Read the model definition and answer for the solid it produces. Units are mm, in the model's axes. Face numbers are marked on the shaded views. A direction names the side the tool comes from. Coordinates: 2 decimals unless noted, no trailing zeros. Loops run counter-clockwise (first coordinate to the right, second up) from the corner with the lowest first, then second, coordinate; pieces in that order, holes last. Notation, with made-up numbers: (80.25, 26) -> (109.25, 26) arc R22 cw to (109.25, 53) -> close; hole circle Ø3 at (85.5, -27). An arc over 180 degrees is marked (long way). Answer as CSV lines item,"result".
Autodesk Inventor part; units mm, degrees
ref_plane "YZ Plane" through (0, 0, 0) normal (1, 0, 0) x (0, 1, 0)
ref_plane "XZ Plane" through (0, 0, 0) normal (0, 1, 0) x (-1, 0, 0)
ref_plane "XY Plane" through (0, 0, 0) normal (0, 0, 1) x (1, 0, 0)
sketch "Sketch1" plane through (0, 0, 0) normal (0, 0, 1) x (1, 0, 0)
  circle A0 centre (0, 0) radius 19
  dimension "d0" = 38
extrude "Base_Shell" add sketch "Sketch1" along normal mid plane 132
sketch "Sketch2" plane through (0, 0, 66) normal (0, 0, 1) x (1, 0, 0)
  circle A0 centre (0, 0) radius 8.75
  dimension "d3" = 17.5
extrude "Terminal_Shell" add sketch "Sketch2" along normal blind 3.8
sketch "Sketch3" plane through (0, 0, 69.8) normal (0, 0, 1) x (1, 0, 0)
  circle A0 centre (0, 0) radius 7.75
  dimension "d6" = 15.5
extrude "Terminal" add sketch "Sketch3" along normal blind 3
sketch "Sketch4" plane through (0, 0, 72.8) normal (0, 0, 1) x (1, 0, 0)
  circle A0 centre (0, 0) radius 2.5
  dimension "d9" = 5
extrude "M5_Terminal_Screw_hole" cut sketch "Sketch4" against normal blind 5
mirror "Mirror1" about plane through (0, 0, 0) normal (0, 0, 1) of "Terminal_Shell", "Terminal", "M5_Terminal_Screw_hole"
equation "\"d1\" = 3.47368 * d0"
equation "\"d3\" = 0.460526 * d0"
equation "\"d4\" = 0.1 * d0"
equation "\"d6\" = 0.407895 * d0"
equation "\"d7\" = 0.0789474 * d0"
equation "\"d9\" = 0.131579 * d0"
equation "\"d10\" = d9"
properties part number "38120s-10Ah" material "Nickel-Copper Alloy 400"
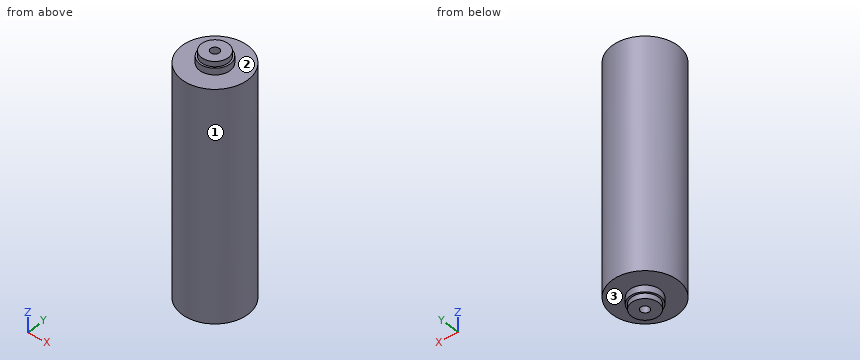
Q1. A cutting plane is placed at C-C, the plane z = -44. Write down the section's boundary in (x, y).
Results:
outline,"circle Ø38 at (0, 0)"
Q2. A cutting plane is placed at D-D, the plane y = -12. Write down the section's boundary in (x, z).
Results:
outline,"(-14.73, -66) -> (14.73, -66) -> (14.73, 66) -> (-14.73, 66) -> close"
Q3. A cutting plane is placed at A-A, the plane x = 0. Write down the section's boundary in (y, z), and give its area (3 significant figures).
Results:
outline,"(-19, -66) -> (-8.75, -66) -> (-8.75, -69.8) -> (-7.75, -69.8) -> (-7.75, -72.8) -> (-2.5, -72.8) -> (-2.5, -67.8) -> (2.5, -67.8) -> (2.5, -72.8) -> (7.75, -72.8) -> (7.75, -69.8) -> (8.75, -69.8) -> (8.75, -66) -> (19, -66) -> (19, 66) -> (8.75, 66) -> (8.75, 69.8) -> (7.75, 69.8) -> (7.75, 72.8) -> (2.5, 72.8) -> (2.5, 67.8) -> (-2.5, 67.8) -> (-2.5, 72.8) -> (-7.75, 72.8) -> (-7.75, 69.8) -> (-8.75, 69.8) -> (-8.75, 66) -> (-19, 66) -> close"
area,"5,190 mm²"
Q4. Given pin 1 Ø4 at (x, y) = (0, 0) entering from -Z; pin 2 Ø6 at (x, z) = (-2, 17.5) entering from -Y; pin 3 Ø4 at (x, z) = (13.5, 8.5) entering from +Y, each flat-ended and moving along its own axis, determine where each tip first touches the part or whether it passes through.
Results:
pin 1,"stops at z = -67.8"
pin 2,"stops at y = -19"
pin 3,"stops at y = 15.12"
Q5. For the marked faces 1, 2 and 3, determine the directions among +Z, -Z, +X, -X, +Y, -Y from which every point of the face is accessible in a straight line to the end or side of a thin tool.
Results:
face 1,"+Z, -Z"
face 2,"+Z"
face 3,"-Z"
Q6. Find the intervals of material crossed by probe 1 along Y at (x, z) = (0, 69); probe 2 along Z at (x, y) = (-10.5, -7.5); probe 3 along Y at (x, z) = (0, 70.15), in increasing order. Write a range as [from, to].
Results:
probe 1,"y = [-8.75, -2.5], [2.5, 8.75]"
probe 2,"z = [-66, 66]"
probe 3,"y = [-7.75, -2.5], [2.5, 7.75]"
